```python
from build123d import *

# Parameters (mm, degrees)
F0_W     = 15
F0_H     = 3.5
F2_R     = 6
F3_DEPTH = 50
F5_DEPTH = 25


with BuildPart() as f1:
    # F0 (on Front) → F1 (revolve)
    with BuildSketch(Plane.XZ):
        with BuildLine():
            Line((62, 12.5), (23.291562, 12.5))
            ThreePointArc((23.291562, 12.5), (7.906814, 13.21691), (0, 0))
            Line((0, 0), (62, 0))
            Line((62, 0), (62, 12.5))
        make_face()
        Polygon((80, 7.5), (62, 12.5), (62, 0), (80, 0), align=None)
        Polygon((95, 7.5), (80, 7.5), (80, 0), (95, 0), (95, 3.5), align=None)
        with Locations((102.5, 1.75)):
            Rectangle(F0_W, F0_H)
    revolve(axis=Axis((60.8708, 0, 0), (1, 0, 0)))

    # F2 (on Front) → F3 (cut, symmetric)
    with BuildSketch(Plane.XZ):
        with Locations((15, 0)):
            Circle(F2_R)
    extrude(amount=F3_DEPTH, both=True, mode=Mode.SUBTRACT)

    # F4 (on Top) → F5 (cut, symmetric)
    with BuildSketch(Plane.XY):
        Polygon((0, -10.235786), (0, 0), (0, 9.764214), (74.575491, 9.764214), (74.575491, 15), (-74.575491, 15), (-74.575491, -15), (74.575491, -15), (74.575491, -10.235786), align=None)
    extrude(amount=F5_DEPTH, both=True, mode=Mode.SUBTRACT)


solid = f1.part
```
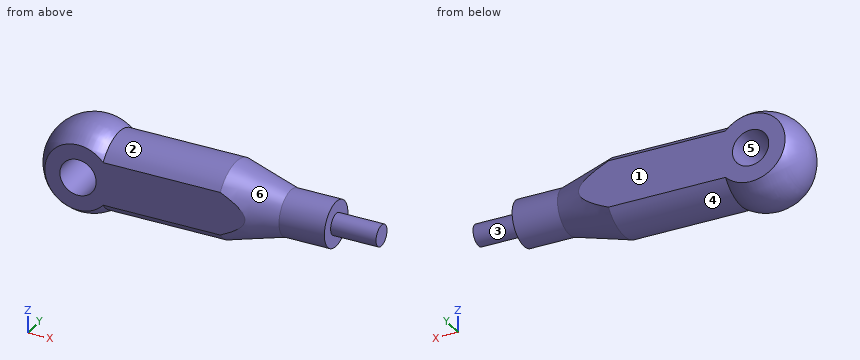
The model under review builds one solid part; all positions refer to its coordinate system, in mm. Face numbers are marked on the shaded views. A direction names the side the tool comes from. Round coordinates to 2 decimals unless told otherwise and drop trailing zeros. Write each loop counter-clockwise with the first axis right and the second up, starting at its lowest first coordinate (ties: lowest second). Pieces come first, ordered by that corner, then holes.
(1) Wall thickness on L1, parallel to Z at x = 15, y = 0.75; L2, parallel to X at y = -3.5, z = -5.5; L3, parallel to Z at x = 44, y = 0.25: over which ranges is each line inside the solid? List them lowest first.
(2) Insertion check: pin 1 (8 mm diameter, centred on x = 47.5, y = 2, fed in from +Z); pin 2 (4 mm diameter, centred on x = 22, y = -4.5, fed in from +Z); pin 3 (11 mm diameter, centred on x = 15, z = 0, fed in from -Y); pin 4 (2 mm diameter, centred on x = 19, y = 0, fed in from -Z). Each pin has a flat end and moves straight along its axis. Give the tip position at first contact, or say it passes through.
(3) We need section A-A on x = 73. Give the boundary of the cut face in (y, z).
(4) Mouldability with a two-part tool opening along X and no side actions: class the marked faces 4, 5 and 6 as +X half, -X half, draft (parallel to the pull), parting line (faces both ways), or undercut.
(5) We need section B-B on x = 36. Give the boundary of the cut face in (y, z).
(6) Machinability: for the marked faces 1, 2 and 3, which of the approach directions +Z, -Z, +X, -X, +Y, -Y give a long, thin tool a straight path to every point of the face, cutting with its end or side? Answer none if there is none.
Findings below:
1. L1: z = -14.98 to -6, 6 to 14.98
1. L2: x = 1.49 to 12.6, 17.4 to 95
1. L3: z = -12.5 to 12.5
2. pin 1: stops at z = 12.5
2. pin 2: stops at z = 13.6
2. pin 3: passes through
2. pin 4: stops at z = -14.7
3. outline: circle Ø18.89 at (0, 0)
4. face 4: draft
4. face 5: undercut
4. face 6: +X half
5. outline: (-10.24, -7.17) arc R12.5 ccw to (9.76, -7.8) - (9.76, 7.8) arc R12.5 ccw to (-10.24, 7.17) - close
6. face 1: +Z, -Z, +X, -X, +Y
6. face 2: +Z, +X
6. face 3: +X
